Geometry: see drawing. Coordinates: mm, zero at the bounding-box minimum. A direction names the side the tool comes from. Coordinates: 2 decimals unless noted, no trailing zeros. Order: outer loops, then holes, each group sorted by start corner. A loop starts at its lowest first (then second) coordinate and runs counter-clockwise, first axis right, second up. Notation, with made-up numbers: (65.5, -6) -> (69.5, -6) arc R18 cw to (69.5, 13) -> close; hole circle Ø10 at (71.25, 80). An arc over 180 degrees is marked (long way). Use CSV: the item, a comma, the result in double quotes. Start each with the question number.
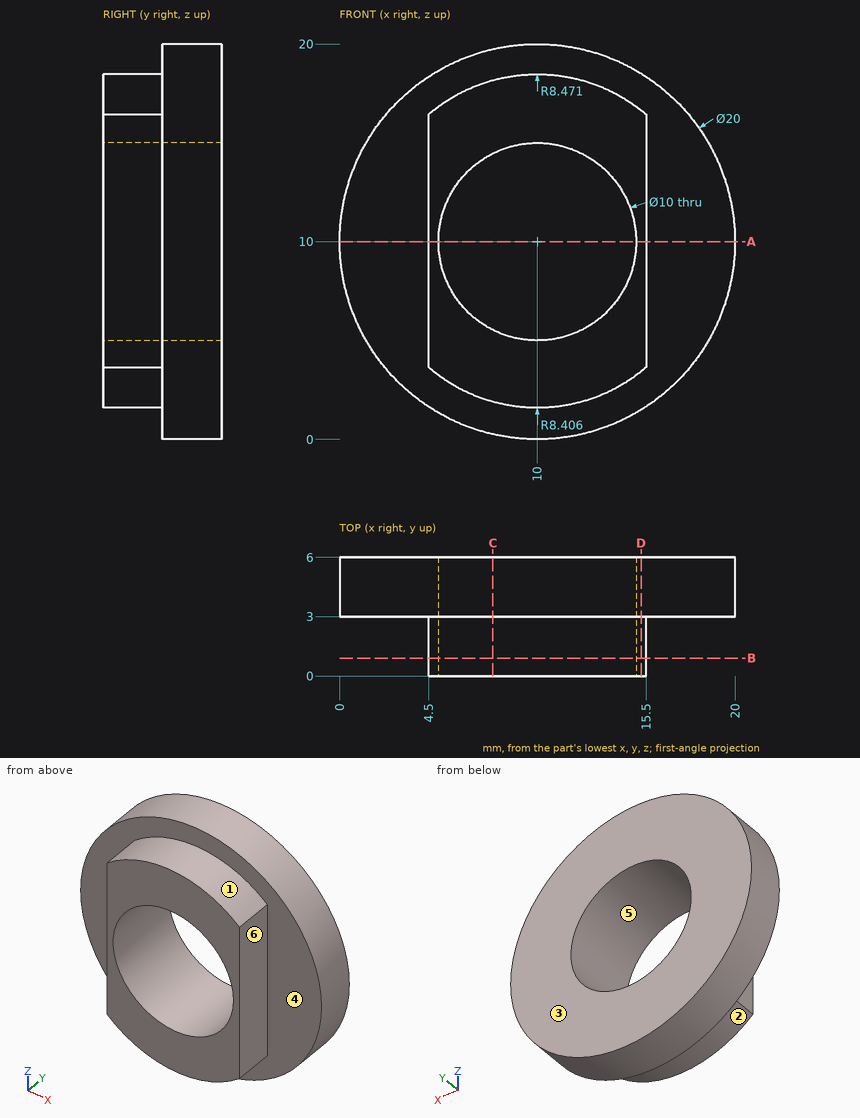
(1) Section C-C (x = 7.75). Return loops of the section in (y, z) (1 decimal).
(2) Access query for the marked faces 1, 2 and 3. Directions: +Z, -Z, +X, -X, +Y, -Y. A direction counts if a zero-diameter tool reaches every point of the face in a straight line with its end or side. Return the directions, or none.
(3) Section A-A (z = 10). Return loops of the section in (x, y).
(4) Section B-B (y = 0.9). Return loops of the section in (x, z).
(5) Mould query, pull axis X, two halves, no side actions, for the marked faces 4, 5 and 6. Classes: pulls with the +X half, pulls with the -X half, needs draft (parallel to the pull), parting line crosses it, or undercut.
(6) First-contact query: pin 1 (2 mm diameter, centred on x = 16.5, y = 2.5, fed in from +Z); pin 2 (3.5 mm diameter, centred on y = 1.5, z = 7, fed in from -X); pin 3 (3.5 mm diameter, centred on y = 2, z = 11, fed in from +X). Flat tips, straight axial feed; report the tip coordinate or a pass-through.
(7) Line query: line 1 (X direction, y = 3.35, z = 10); line 2 (X direction, y = 1.85, z = 10); line 3 (Z direction, x = 10, y = 2.85). Output: solid intervals per line, ascending. Write a range as from..to.
(8) Section D-D (x = 15.25). Return loops of the section in (y, z) (1 decimal).
Check sheet entries:
1,outline,"(0, 1.9) -> (3, 1.9) -> (3, 0.3) -> (6, 0.3) -> (6, 5.5) -> (0, 5.5) -> close; (0, 14.5) -> (6, 14.5) -> (6, 19.7) -> (3, 19.7) -> (3, 18.2) -> (0, 18.2) -> close"
2,face 1,"+Z, -Y"
2,face 2,"-Z, -Y"
2,face 3,"+Z, -Z, +X, -X, +Y"
3,outline,"(0, 3) -> (4.5, 3) -> (4.5, 0) -> (5, 0) -> (5, 6) -> (0, 6) -> close; (15, 0) -> (15.5, 0) -> (15.5, 3) -> (20, 3) -> (20, 6) -> (15, 6) -> close"
4,outline,"(4.5, 3.64) arc R8.41 ccw to (15.5, 3.64) -> (15.5, 16.44) arc R8.47 ccw to (4.5, 16.44) -> close; hole circle Ø10 at (10, 10)"
5,face 4,"needs draft"
5,face 5,"undercut"
5,face 6,"pulls with the +X half"
6,pin 1,"stops at z = 18.26"
6,pin 2,"stops at x = 0.22"
6,pin 3,"stops at x = 20"
7,line 1,"x = 0..5, 15..20"
7,line 2,"x = 4.5..5, 15..15.5"
7,line 3,"z = 1.59..5, 15..18.47"
8,outline,"(0, 3.4) -> (3, 3.4) -> (3, 1.5) -> (6, 1.5) -> (6, 18.5) -> (3, 18.5) -> (3, 16.6) -> (0, 16.6) -> close"
